Verification items for the finished model (mm, model axes). A direction names the side the tool comes from. Coordinates: 2 decimals unless noted, no trailing zeros. Write each loop counter-clockwise with the first axis right and the second up, starting at its lowest first coordinate (ties: lowest second). Pieces come first, ordered by that corner, then holes. Notation, with made-up numbers: (44, -10.75) -> (50, -10.75) arc R11 cw to (50, -4.75) -> close; hole circle Ø4 at (77.25, 64). An arc over 180 degrees is marked (long way). Use CSV: the item, a comma, the result in double quotes.
Autodesk Inventor part; units mm, degrees
ref_plane "YZ Plane" through (0, 0, 0) normal (1, 0, 0) x (0, 1, 0)
ref_plane "XZ Plane" through (0, 0, 0) normal (0, 1, 0) x (-1, 0, 0)
ref_plane "XY Plane" through (0, 0, 0) normal (0, 0, 1) x (1, 0, 0)
sketch "Sketch1" plane through (0, 0, 0) normal (0, 0, 1) x (1, 0, 0)
  circle A0 centre (0, 4.7625) radius 3.175
  arc A1 (-7.9074, -0.6902) -> (7.9074, -0.6902) centre (0, 0) ccw
  line L0 (3.175, 4.7625) -> (3.175, 0.635)
  line L1 (3.81, 0) -> (7.2748, 0)
  line L2 (-3.175, 4.7625) -> (-3.175, 0.635)
  line L3 (-3.81, 0) -> (-7.2748, 0)
  arc A2 (-7.2748, 0) -> (-7.9074, -0.6902) centre (-7.2748, -0.635) ccw
  arc A3 (-3.81, 0) -> (-3.175, 0.635) centre (-3.81, 0.635) ccw
  arc A4 (3.175, 0.635) -> (3.81, 0) centre (3.81, 0.635) ccw
  arc A5 (7.9074, -0.6902) -> (7.2748, 0) centre (7.2748, -0.635) ccw
  circle A6 centre (0, 0) radius 3.175
  circle A7 centre (0, 4.7625) radius 3.175
  point P0 (-3.175, 0)
  point P1 (-7.9375, 0)
  point P2 (7.9375, 0)
  dimension "d2" = 0.635
  dimension "d3" = 0.635
  dimension "d4" = 6.35
extrude "Extrusion1" add sketch "Sketch1" along normal blind 12.7 contours A6 A0 | A0 A6 picked at (-0.105, -1.5684) picked at (-0.2525, 2.1472)
extrude "Extrusion2" add sketch "Sketch1" against normal blind 3.175
extrude "Extrusion3" add sketch "Sketch1" against normal blind 12.7 contours A0 A6 | A0 A6 picked at (0, 6.3346) picked at (-0.2525, 2.1472)
properties part number "Crankshaft"
1) Scan lines: L1, parallel to Z at x = 5.5, y = -5 (3 decimals); L2, parallel to Z at x = 2, y = 4.5; L3, parallel to Y at x = 1.25, z = -3.5. Record each from-to range of solid material in increasing order.
Return value:
L1,"-3.175 to 0"
L2,"-12.7 to 0"
L3,"1.84 to 7.68"
2) Cross-section at A-A (x = 0). Record the boundary of the cut face in (y, z) (1 decimal).
Return value:
outline,"(-7.9, -3.2) -> (1.6, -3.2) -> (1.6, -12.7) -> (7.9, -12.7) -> (7.9, 0) -> (3.2, 0) -> (3.2, 12.7) -> (-3.2, 12.7) -> (-3.2, 0) -> (-7.9, 0) -> close"
3) Set-up check for faces 1 (the cylindrical face through (-0.69, 3.1, 6.26)), 2 (the flat face through (3.175, 3, -2)), 3 (the flat face through (-3.175, 3, -2)): record each of +Z, -Z, +X, -X, +Y, -Y from which the full face is reachable in a straight line by a thin tool's end or side.
Return value:
face 1,"+Z"
face 2,"+Z, -Z, +X, +Y"
face 3,"+Z, -Z, -X, +Y"
4) Cross-section at B-B (y = 2.5). Record the boundary of the cut face in (x, z) (1 decimal), plus the area to 3 significant figures.
Return value:
outline,"(-3.2, -3.2) -> (-2.2, -3.2) -> (-2.2, -12.7) -> (2.2, -12.7) -> (2.2, -3.2) -> (3.2, -3.2) -> (3.2, 0) -> (2, 0) -> (2, 12.7) -> (-2, 12.7) -> (-2, 0) -> (-3.2, 0) -> close"
area,"112 mm2"
5) Cross-section at D-D (x = -5.75). Record the boundary of the cut face in (y, z) (3 decimals).
Return value:
outline,"(-5.472, -3.175) -> (0, -3.175) -> (0, 0) -> (-5.472, 0) -> close"
6) Gauge pin test, flat ends, axial feed: pin 1 (8 mm diameter, centred on x = -6, z = 2.5, fed in from -Y); pin 2 (6.5 mm diameter, centred on x = 0.5, y = -2, fed in from -Z) (3 decimals); pin 3 (3 mm diameter, centred on x = -5.5, y = 5.5, fed in from -Z); pin 4 (3.5 mm diameter, centred on y = 3, z = -2.5, fed in from +X) (3 decimals). Record the tip position at first contact, or that the pin passes through.
Return value:
pin 1,"y = -7.4"
pin 2,"z = -3.175"
pin 3,"through"
pin 4,"x = 3.175"
